Input: dimensioned drawing with shaded views. Units: mm. Origin: part minimum x, y, z. A direction names the side the tool comes from. Round coordinates to 2 decimals unless told otherwise and drop trailing zeros. Order: outer loops, then holes, each group sorted by start corner. A loop starts at its lowest first (then second) coordinate and runs counter-clockwise, first axis right, second up. Notation, with made-up numbers: (67.5, -18.75) -> (87.5, -18.75) arc R31 cw to (87.5, 11.25) -> close; hole circle Ø11 at (48, -39). An arc over 180 degrees is marked (long way). Use a Markdown table: item, result. Add a question column.
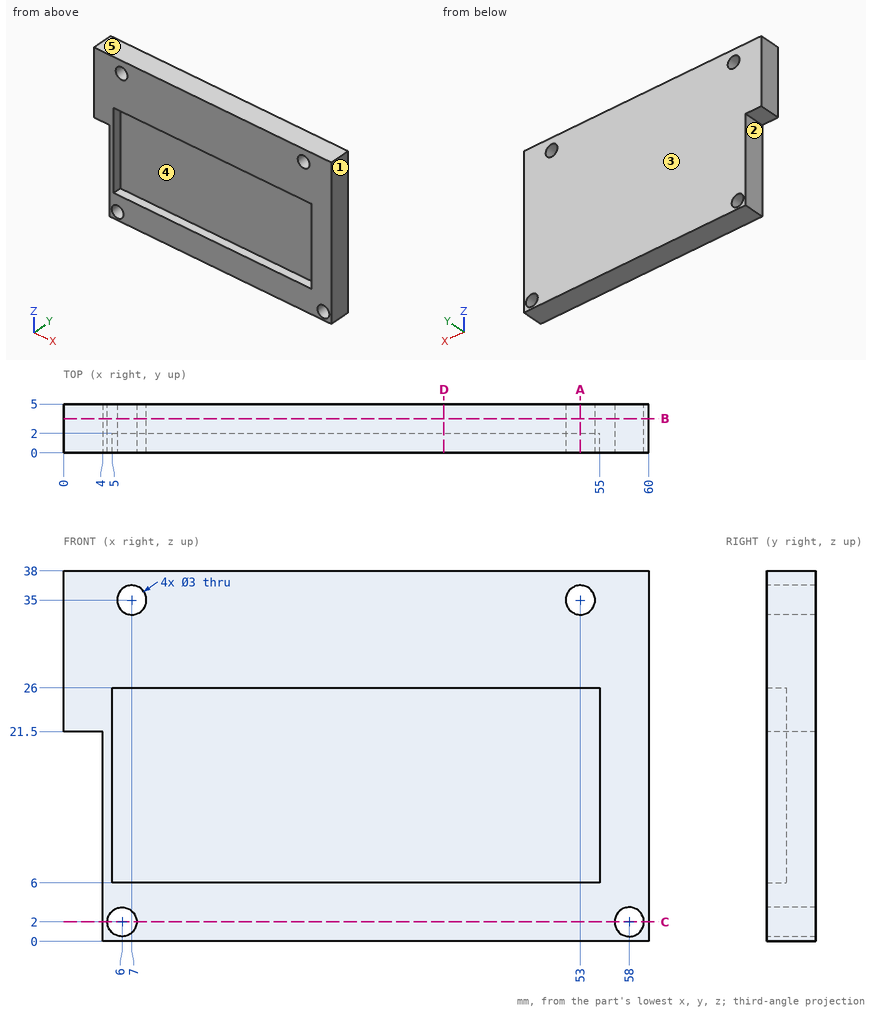
1) Draft query along Z for the marked faces 3, 4 and 5. Return one class per face: pulls with the +Z half, pulls with the -Z half, needs draft (parallel to the pull), parting line crosses it, or undercut.
2) Section C-C on z = 2. Output: boundary loops of the cut face in (x, y).
3) Section D-D on x = 39. Output: boundary loops of the cut face in (y, z), then the cut area to 3 significant figures.
4) Section B-B on y = 3.5. Output: boundary loops of the cut face in (x, z), then the cut area to 3 significant figures.
5) Section A-A on x = 53. Output: boundary loops of the cut face in (y, z), then the cut area to 3 significant figures.
6) First-contact query: pin 1 Ø1.8 at (x, z) = (7, 35) entering from -Y; pin 2 Ø0.6 at (y, z) = (0.5, 11.5) entering from -X; pin 3 Ø1.5 at (x, z) = (12.5, 20) entering from -Y; pin 4 Ø1.2 at (x, y) = (2.5, 2.5) entering from -Z. Flat tips, straight axial feed; report the tip coordinate or a pass-through.
7) Reachability of the marked faces 1 and 2 from +Z, -Z, +X, -X, +Y, -Y: full face, straight path, thin tool, end or side. Return the list, or none.
8) Line query: probe 1 along X at (y, z) = (0.6, 19); probe 2 along Z at (x, y) = (12, 1.9); probe 3 along Z at (x, y) = (6, 3.6). Output: solid intervals per line, ascending. Write a range as from..to.
Conclusion:
| question | item | result |
|---|---|---|
| 1 | face 3 | needs draft |
| 1 | face 4 | undercut |
| 1 | face 5 | pulls with the +Z half |
| 2 | outline | (4, 0) -> (4.5, 0) -> (4.5, 5) -> (4, 5) -> close; (7.5, 0) -> (56.5, 0) -> (56.5, 5) -> (7.5, 5) -> close; (59.5, 0) -> (60, 0) -> (60, 5) -> (59.5, 5) -> close |
| 3 | outline | (0, 0) -> (5, 0) -> (5, 38) -> (0, 38) -> (0, 26) -> (2, 26) -> (2, 6) -> (0, 6) -> close |
| 3 | area | 150 mm^2 |
| 4 | outline | (0, 21.5) -> (4, 21.5) -> (4, 0) -> (60, 0) -> (60, 38) -> (0, 38) -> close; hole circle Ø3 at (6, 2); hole circle Ø3 at (7, 35); hole circle Ø3 at (53, 35); hole circle Ø3 at (58, 2) |
| 4 | area | 2,170 mm^2 |
| 5 | outline | (0, 0) -> (5, 0) -> (5, 33.5) -> (0, 33.5) -> (0, 26) -> (2, 26) -> (2, 6) -> (0, 6) -> close; (0, 36.5) -> (5, 36.5) -> (5, 38) -> (0, 38) -> close |
| 5 | area | 135 mm^2 |
| 6 | pin 1 | passes through |
| 6 | pin 2 | stops at x = 4 |
| 6 | pin 3 | stops at y = 2 |
| 6 | pin 4 | stops at z = 21.5 |
| 7 | face 1 | +Z, -Z, +X, +Y, -Y |
| 7 | face 2 | -Z, -X, +Y, -Y |
| 8 | probe 1 | x = 4..5, 55..60 |
| 8 | probe 2 | z = 0..6, 26..38 |
| 8 | probe 3 | z = 0..0.5, 3.5..33.88, 36.12..38 |
